from build123d import *

# Parameters (mm, degrees)
MOTOR_SUPPORT_FRONT_PADDLE_MASTER_2_W = 30.52
MOTOR_SUPPORT_FRONT_PADDLE_MASTER_2_H = 109.191376887
MOTOR_SUPPORT_FRONT_PADDLE_MASTER_2_R = 1.5
BOSS_EXTRUDE1_DEPTH                   = 4.11
CUT_EXTRUDE1_START                    = -37.61
SKETCH14_PADDLE_MASTER_2_W            = 4.11
SKETCH14_PADDLE_MASTER_2_H            = 6
CUT_EXTRUDE1_DEPTH                    = 4.11
PADDLE_MASTER_START                   = -5
PADDLE_MASTER_OUTLINE_W               = 4.11
PADDLE_MASTER_OUTLINE_H               = 4.11
PADDLE_MASTER_DEPTH                   = 10


# Read off the part's stored shape, not the designer's step: paddle_master
with BuildPart() as part:
    # motor_support_front-paddle_master<2> → Boss-Extrude1 (new body)
    with BuildSketch(Plane(origin=(0, -2.5, 5), x_dir=(1, 0, 0), z_dir=(0, 0, 1))):
        with Locations((0, -66.737824068)):
            Rectangle(MOTOR_SUPPORT_FRONT_PADDLE_MASTER_2_W, MOTOR_SUPPORT_FRONT_PADDLE_MASTER_2_H)
        with Locations((8.5, -17.73)):
            Circle(MOTOR_SUPPORT_FRONT_PADDLE_MASTER_2_R, mode=Mode.SUBTRACT)
        with Locations((-8.5, -17.73)):
            Circle(MOTOR_SUPPORT_FRONT_PADDLE_MASTER_2_R, mode=Mode.SUBTRACT)
    extrude(amount=-BOSS_EXTRUDE1_DEPTH)

    # Sketch14-paddle_master<2> → Cut-Extrude1 (cut)
    with BuildSketch(Plane(origin=(11.15, 12.5, 38.5), x_dir=(1, 0, 0), z_dir=(0, 0, 1)).offset(CUT_EXTRUDE1_START)):
        with Locations((-24.355, -125.223512511)):
            Rectangle(SKETCH14_PADDLE_MASTER_2_W, SKETCH14_PADDLE_MASTER_2_H)
        with Locations((-24.355, -115.223512511)):
            Rectangle(SKETCH14_PADDLE_MASTER_2_W, SKETCH14_PADDLE_MASTER_2_H)
        with Locations((-24.355, -105.223512511)):
            Rectangle(SKETCH14_PADDLE_MASTER_2_W, SKETCH14_PADDLE_MASTER_2_H)
        with Locations((2.055, -125.223512511)):
            Rectangle(SKETCH14_PADDLE_MASTER_2_W, SKETCH14_PADDLE_MASTER_2_H)
        with Locations((2.055, -115.223512511)):
            Rectangle(SKETCH14_PADDLE_MASTER_2_W, SKETCH14_PADDLE_MASTER_2_H)
        with Locations((2.055, -105.223512511)):
            Rectangle(SKETCH14_PADDLE_MASTER_2_W, SKETCH14_PADDLE_MASTER_2_H)
    extrude(amount=CUT_EXTRUDE1_DEPTH, mode=Mode.SUBTRACT)

    # paddle_master outline → paddle_master (cut)
    with BuildSketch(Plane.YZ.offset(PADDLE_MASTER_START)):
        with Locations((-121.778512511, 2.945)):
            Rectangle(PADDLE_MASTER_OUTLINE_W, PADDLE_MASTER_OUTLINE_H)
    extrude(amount=PADDLE_MASTER_DEPTH, mode=Mode.SUBTRACT)


solid = part.part
CAD build for the part. Positions are in the model's coordinates, mm. A direction names the side the tool comes from. Round coordinates to 2 decimals unless told otherwise and drop trailing zeros. Order: outer loops, then holes, each group sorted by start corner. A loop starts at its lowest first (then second) coordinate and runs counter-clockwise, first axis right, second up. Notation, with made-up numbers: (60.5, 12.5) - (100.5, 12.5) arc R15 cw to (100.5, 39.5) - close; hole circle Ø1 at (-37.5, -12.75). An arc over 180 degrees is marked (long way). Return JSON: item names as keys, results as strings.
(1) Pull direction X, two halves, no side cores. Call faces 1 (the face through (5, -122, 3)), 2 (the face through (10, -123.834, 3)), 3 (the face through (-15.26, -120, 3)): +X half, -X half, draft (parallel to the pull), parting line (faces both ways), or undercut.
Answer key:
{"face 1": "undercut", "face 2": "draft", "face 3": "-X half"}
(2) Cut at A-A (x = -8.5). Give the cut face in (y, z).
Answer key:
{"outline": "(-123.83, 0.89) - (-21.73, 0.89) - (-21.73, 5) - (-123.83, 5) - close; (-18.73, 0.89) - (-14.64, 0.89) - (-14.64, 5) - (-18.73, 5) - close"}
(3) Wall check: probe 1 along Y at (x, z) = (13, 4.05); probe 2 along Y at (x, z) = (8.5, 1.9); probe 3 along Y at (x, z) = (-2, 4.1). Give the ranges that are in metal, low to high. Write a range as from..to.
Answer key:
{"probe 1": "y = -123.83..-115.72, -109.72..-105.72, -99.72..-95.72, -89.72..-14.64", "probe 2": "y = -123.83..-21.73, -18.73..-14.64", "probe 3": "y = -119.72..-14.64"}
(4) Cut at B-B (z = 2.55). State how many separate pieces and enclosed holes the cut face has, then the cut area to 3 significant figures.
Answer key:
{"separate pieces": "1", "enclosed holes": "2", "area": "3,130 mm^2"}
(5) Tool access for faces 4 (the face through (-15.26, -98, 3)), 5 (the face through (13, -99.724, 3)), 6 (the face through (-13, -115.724, 3)): list every direction of +Z, -Z, +X, -X, +Y, -Y with a clear straight run to the whole face (end or side of a thin tool).
Answer key:
{"face 4": "+Z, -Z, -X, +Y, -Y", "face 5": "+Z, -Z, +X", "face 6": "+Z, -Z, -X"}
(6) Cut at C-C (y = -20.23). Give the cut face in (x, z), then the cut area to 3 significant figures.
Answer key:
{"outline": "(-15.26, 0.89) - (-10, 0.89) - (-10, 5) - (-15.26, 5) - close; (-7, 0.89) - (7, 0.89) - (7, 5) - (-7, 5) - close; (10, 0.89) - (15.26, 0.89) - (15.26, 5) - (10, 5) - close", "area": "101 mm^2"}
(7) Pin check, flat tips, straight feed: pin 1 Ø2 at (y, z) = (-112.5, 4) entering from +X; pin 2 Ø1.2 at (y, z) = (-113, 3.5) entering from -X; pin 3 Ø2.5 at (x, y) = (-8.5, -20.23) entering from +Z. Stop position of each tip, or through.
Answer key:
{"pin 1": "stops at x = 11.15", "pin 2": "stops at x = -11.15", "pin 3": "passes through"}
